```python
from build123d import *

# Parameters (mm, degrees)
F0_R     = 11.2
F1_DEPTH = 7
F2_R     = 1.5
F3_R     = 1.5


with BuildPart() as f1:
    # F0 (on Top) → F1 (new body)
    with BuildSketch(Plane.XY):
        with BuildLine():
            Line((7.7504207738, -16.3618978113), (11.378000875, -10.0787447675))
            ThreePointArc((11.378000875, -10.0787447675), (13.1635861375, -7.6), (14.4174494444, -4.8142654183))
            Line((14.4174494444, -4.8142654183), (18.0450295456, 1.4688876255))
            Line((18.0450295456, 1.4688876255), (38.6342470892, 1.4688876255))
            ThreePointArc((38.6342470892, 1.4688876255), (26.5584523993, 12.6016397781), (10.2946087718, 14.8930101858))
            Line((10.2946087718, 14.8930101858), (3.0394485694, 14.8930101858))
            Line((3.0394485694, 14.8930101858), (-3.0394485694, 14.8930101858))
            Line((-3.0394485694, 14.8930101858), (-10.2946087718, 14.8930101858))
            Line((-10.2946087718, 14.8930101858), (-20.5892175436, 32.7237956226))
            ThreePointArc((-20.5892175436, 32.7237956226), (-24.1925663768, 16.6994745739), (-18.0450295456, 1.4688876255))
            Line((-18.0450295456, 1.4688876255), (-7.7504207738, -16.3618978113))
            Line((-7.7504207738, -16.3618978113), (-18.0450295456, -34.1926832481))
            ThreePointArc((-18.0450295456, -34.1926832481), (-2.3658860225, -29.301114352), (7.7504207738, -16.3618978113))
        make_face()
        Circle(F0_R, mode=Mode.SUBTRACT)
        Polygon((-38.6342470892, -34.1926832481), (-18.0450295456, -34.1926832481), (-7.7504207738, -16.3618978113), (-18.0450295456, 1.4688876255), (-38.6342470892, 1.4688876255), (-48.928855861, -16.3618978113), align=None)
        with Locations((-28.3396383174, -16.3618978113)):
            Circle(F0_R, mode=Mode.SUBTRACT)
        with BuildLine():
            ThreePointArc((14.4174494444, -4.8142654183), (13.1635861375, -7.6), (11.378000875, -10.0787447675))
            Line((11.378000875, -10.0787447675), (7.7504207738, -16.3618978113))
            Line((7.7504207738, -16.3618978113), (18.0450295456, -34.1926832481))
            Line((18.0450295456, -34.1926832481), (38.6342470892, -34.1926832481))
            Line((38.6342470892, -34.1926832481), (48.928855861, -16.3618978113))
            Line((48.928855861, -16.3618978113), (38.6342470892, 1.4688876255))
            Line((38.6342470892, 1.4688876255), (18.0450295456, 1.4688876255))
            Line((18.0450295456, 1.4688876255), (14.4174494444, -4.8142654183))
        make_face()
        with Locations((28.3396383174, -16.3618978113)):
            Circle(F0_R, mode=Mode.SUBTRACT)
        Polygon((3.0394485694, 14.8930101858), (10.2946087718, 14.8930101858), (20.5892175436, 32.7237956226), (10.2946087718, 50.5545810594), (-10.2946087718, 50.5545810594), (-20.5892175436, 32.7237956226), (-10.2946087718, 14.8930101858), (-3.0394485694, 14.8930101858), align=None)
        with Locations((0, 32.7237956226)):
            Circle(F0_R, mode=Mode.SUBTRACT)
    extrude(amount=F1_DEPTH)

    # F2
    f2_edges = [f1.edges().sort_by_distance(p)[0] for p in [
        (-24.192566, 16.699475, 7),
        (-15.441913, 41.639188, 7),
        (0, 50.554581, 7),
        (15.441913, 41.639188, 7),
        (15.441913, 23.808403, 7),
        (26.558452, 12.60164, 7),
        (43.781551, -7.446505, 7),
        (43.781551, -25.277291, 7),
        (28.339638, -34.192683, 7),
        (12.897725, -25.277291, 7),
        (-2.365886, -29.301114, 7),
        (-28.339638, -34.192683, 7),
        (-43.781551, -25.277291, 7),
        (-43.781551, -7.446505, 7),
        (-28.339638, 1.468888, 7),
    ]]
    fillet(f2_edges, radius=F2_R)

    # F3
    f3_edges = [f1.edges().sort_by_distance(p)[0] for p in [
        (-28.339638, -34.192683, 0),
        (-2.365886, -29.301114, 0),
        (12.897725, -25.277291, 0),
        (28.339638, -34.192683, 0),
        (43.781551, -25.277291, 0),
        (43.781551, -7.446505, 0),
        (26.558452, 12.60164, 0),
        (15.441913, 23.808403, 0),
        (15.441913, 41.639188, 0),
        (0, 50.554581, 0),
        (-15.441913, 41.639188, 0),
        (-24.192566, 16.699475, 0),
        (-28.339638, 1.468888, 0),
        (-43.781551, -7.446505, 0),
        (-43.781551, -25.277291, 0),
    ]]
    fillet(f3_edges, radius=F3_R)


solid = f1.part
```
Could you check a few things on this model? Use its own coordinates, in mm. A direction names the side the tool comes from. Round coordinates to 2 decimals unless told otherwise and drop trailing zeros. Loops run counter-clockwise (first coordinate to the right, second up) from the corner with the lowest first, then second, coordinate; pieces in that order, holes last. Notation, with made-up numbers: (51.5, 37.5) -> (57.5, 37.5) arc R25 ccw to (57.5, 59.5) -> close; hole circle Ø11 at (57.25, -12). An arc over 180 degrees is marked (long way). One line per question, with ' | ' between items.
(1) If I drill on probe 1 along Y at (x, z) = (-4.5, 6); probe 2 along Y at (x, z) = (0, 1.5); probe 3 along X at (y, z) = (-19, 6.75), over which ranges is the centre line in solid material (lowest first)?
Model answer:
probe 1: y = -30.54 to -10.26, 10.26 to 22.47, 42.98 to 50.47 | probe 2: y = -27.47 to -11.2, 11.2 to 21.52, 43.92 to 50.55 | probe 3: x = -46.63 to -39.22, -17.45 to 5.84, 10.05 to 17.45, 39.22 to 46.63
(2) If we section it at B-B on y = -18: Count the separate pieces of the cut face and the enclosed holes in it, and give its area (3 significant figures).
Model answer:
separate pieces: 4 | enclosed holes: 0 | area: 346 mm^2
(3) For faces 5 (the face through (12.51, -23.71, 0.43)), 6 (the face through (0, 50.555, 3)), 7 (the face through (12.826, -25.152, 3.472)), which set-ups out of +Z, -Z, +X, -X, +Y, -Y let a thin tool reach every point of the face, with its end or its side?
Model answer:
face 5: -Z, -Y | face 6: +Z, -Z, +X, -X, +Y | face 7: +Z, -Z, -Y
(4) For pin 1 Ø1.2 at (x, z) = (-26.5, 4.5) entering from +Y; pin 2 Ø4 at (x, z) = (-11, 4) entering from +Y, each with a flat end and sliding along its axis, tell me the tip position at first contact or that it passes through.
Model answer:
pin 1: stops at y = 1.47 | pin 2: stops at y = 50.55
(5) If we section it at A-A on x = -28: List the corners of the cut face in (y, z) for me.
Model answer:
outline: (-34.19, 1.5) arc R1.5 ccw to (-32.69, 0) -> (-27.56, 0) -> (-27.56, 7) -> (-32.69, 7) arc R1.5 ccw to (-34.19, 5.5) -> close; (-5.17, 0) -> (-0.03, 0) arc R1.5 ccw to (1.47, 1.5) -> (1.47, 5.5) arc R1.5 ccw to (-0.03, 7) -> (-5.17, 7) -> close
(6) Thinking about a two-plate mould opening in X: for faces 1 (the face through (-28, 1.469, 3)), 2 (the face through (12.491, -23.718, 6.549)), 3 (the face through (43.463, -24.927, 0.428)), 4 (the face through (-43.32, -25.18, 0.43)), which applies, released by +X, released by -X, zero draft, split by the parting line, or undercut?
Model answer:
face 1: zero draft | face 2: undercut | face 3: released by +X | face 4: released by -X
